Autodesk Inventor part; units mm, degrees
ref_plane "YZ Plane" through (0, 0, 0) normal (1, 0, 0) x (0, 1, 0)
ref_plane "XZ Plane" through (0, 0, 0) normal (0, 1, 0) x (-1, 0, 0)
ref_plane "XY Plane" through (0, 0, 0) normal (0, 0, 1) x (1, 0, 0)
sketch "Sketch1" plane through (0, 0, 0) normal (0, 0, 1) x (1, 0, 0)
  arc A0 (-16.164461, 16.164461) -> (20.718196, -9.661053) centre (0, 0) ccw
  arc A1 (-16.254264, 16.254264) -> (20.833297, -9.714726) centre (0, 0) ccw
  line L0 (-16.254264, 16.254264) -> (-16.164461, 16.164461)
  line L1 (20.718196, -9.661053) -> (20.833297, -9.714726)
  line L2 (0, 0) -> (15.160579, 0) construction
  line L3 (20.718196, -9.661053) -> (23.862711, -2.72013)
  line L4 (23.862711, -2.72013) -> (23.978386, -2.772535)
  line L5 (23.978386, -2.772535) -> (20.833297, -9.714726)
  line L6 (-16.254264, 16.254264) -> (-7.274007, 25.23452)
  line L7 (-7.274007, 25.23452) -> (-7.184205, 25.144717)
  line L8 (-7.184205, 25.144717) -> (-16.164461, 16.164461)
  line L9 (0, 0) -> (0, 16.116809) construction
  dimension "d0" = 45.72
  dimension "d1" = 45.974
  dimension "d2" = 25
  dimension "d3" = 7.62
  dimension "d5" = 12.7
  dimension "d6" = 45
sketch "Sketch1 outline for Extrusion1" plane through (0, 0, 0) normal (0, 0, 1) x (1, 0, 0)
  line L0 (-7.274007, 25.23452) -> (-16.254264, 16.254264)
  arc A0 (-16.254264, 16.254264) -> (20.833297, -9.714726) centre (0, 0) ccw
  line L1 (23.978386, -2.772535) -> (20.833297, -9.714726)
  line L2 (23.862711, -2.72013) -> (23.978386, -2.772535)
  line L3 (20.718196, -9.661053) -> (23.862711, -2.72013)
  arc A1 (20.718196, -9.661053) -> (-16.164461, 16.164461) centre (0, 0) cw
  line L4 (-16.164461, 16.164461) -> (-7.184205, 25.144717)
  line L5 (-7.184205, 25.144717) -> (-7.274007, 25.23452)
extrude "Extrusion1" add sketch "Sketch1 outline for Extrusion1" along normal blind 2.159
properties part number "CopperContact" material "Copper, Alloy"
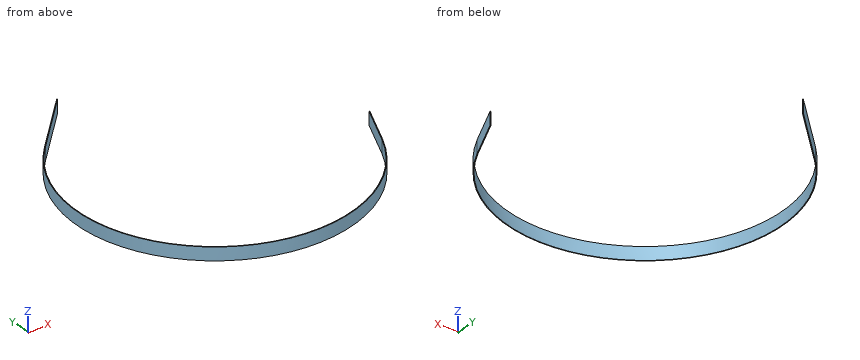
Verification items for the finished model (mm, model axes). Give positions to 0.01 mm unless a question says otherwise; leave off trailing zeros. Write each loop counter-clockwise with the first axis right and the second up, starting at its lowest first coordinate (ties: lowest second). Pieces come first, ordered by that corner, then holes. Notation, with made-up numbers: (-24, 1) -> (-7, 1) arc R12 cw to (-7, 11) -> close; hole circle Ø2 at (-24, 8.5). An arc over 180 degrees is marked (long way). Use CSV: the item, a comma, the result in double quotes.
(1) Sectioned sample at B-B (x = -9). Record the cut outline in (y, z).
Derived:
outline,"(-21.15, 0) -> (-21.01, 0) -> (-21.01, 2.16) -> (-21.15, 2.16) -> close; (23.33, 0) -> (23.51, 0) -> (23.51, 2.16) -> (23.33, 2.16) -> close"
(2) Sectioned sample at A-A (y = -18). Record the cut outline in (x, z).
Derived:
outline,"(-14.3, 0) -> (-14.09, 0) -> (-14.09, 2.16) -> (-14.3, 2.16) -> close; (14.09, 0) -> (14.3, 0) -> (14.3, 2.16) -> (14.09, 2.16) -> close"
(3) Sectioned sample at D-D (y = 0). Record the cut outline in (x, z), plus the area to 3 significant figures.
Derived:
outline,"(-22.99, 0) -> (-22.86, 0) -> (-22.86, 2.16) -> (-22.99, 2.16) -> close"
area,"0.274 mm^2"
(4) Go/stop test with a flat-tipped pin: pin 1 (6 mm diameter, centred on x = -17.5, y = 4, fed in from +Z). Record where the tip stops, or that it passes through.
Derived:
pin 1,"passes through"
(5) Sectioned sample at C-C (z = 0.95). Record the cut outline in (x, y), plus the area to 3 significant figures.
Derived:
outline,"(-16.25, 16.25) arc R22.99 ccw (long way) to (20.83, -9.71) -> (23.98, -2.77) -> (23.86, -2.72) -> (20.72, -9.66) arc R22.86 cw (long way) to (-16.16, 16.16) -> (-7.18, 25.14) -> (-7.27, 25.23) -> close"
area,"12.7 mm^2"
(6) Material ranges on L1, parallel to X at y = -15, z = 1.3; L2, parallel to Y at x = -18.5, z = 0.4; L3, parallel to Y at x = -13, z = 0.4, recorded low to high.
Derived:
L1,"x = -17.42 to -17.25, 17.25 to 17.42"
L2,"y = -13.64 to -13.43, 13.43 to 13.64"
L3,"y = -18.96 to -18.8, 19.33 to 19.51"
